Read the model definition and answer for the solid it produces. Units are mm, in the model's axes. A direction names the side the tool comes from. Give positions to 0.01 mm unless a question says otherwise; leave off trailing zeros. Order: outer loops, then holes, each group sorted by start corner. A loop starts at its lowest first (then second) coordinate and runs counter-clockwise, first axis right, second up.
```python
from build123d import *

# Parameters (mm, degrees)
SKETCH_W        = 56
SKETCH_H        = 45
PAD_DEPTH       = 1
SKETCH001_W     = 53
SKETCH001_H     = 34
PAD001_DEPTH    = 2
SKETCH002_W     = 10
SKETCH002_H     = 5
PAD002_DEPTH    = 4
SKETCH003_R     = 1.7
POCKET_DEPTH    = 38.501
SKETCH004_W     = 6
SKETCH004_H     = 3
POCKET001_DEPTH = 6
FILLET_R        = 4


with BuildPart() as part:
    # Sketch → Pad (new body, symmetric)
    with BuildSketch(Plane.XY):
        with Locations((28, 22.5)):
            Rectangle(SKETCH_W, SKETCH_H)
    extrude(amount=PAD_DEPTH, both=True)

    # Sketch001 (on Face6 of Pad) → Pad001 (join)
    with BuildSketch(Plane.XY.offset(1)):
        with Locations((28, 23.5)):
            Rectangle(SKETCH001_W, SKETCH001_H)
    extrude(amount=PAD001_DEPTH)

    # Sketch002 (on Face11 of Pad001) → Pad002 (join)
    with BuildSketch(Plane.XY.offset(3)):
        with Locations((28, 9)):
            Rectangle(SKETCH002_W, SKETCH002_H)
    extrude(amount=PAD002_DEPTH)

    # Sketch003 (on Face12 of Pad002) → Pocket (cut, through all)
    with BuildSketch(Plane.XZ.offset(-6.5)):
        with Locations((28, 4)):
            Circle(SKETCH003_R)
    extrude(amount=-POCKET_DEPTH, mode=Mode.SUBTRACT)

    # Sketch004 → Pocket001 (cut)
    with BuildSketch(Plane.XY.offset(7)):
        with Locations((28, 9)):
            Rectangle(SKETCH004_W, SKETCH004_H)
    extrude(amount=-POCKET001_DEPTH, mode=Mode.SUBTRACT)

    # Fillet
    fillet_edges = [part.edges().sort_by_distance(p)[0] for p in [
        (0, 0, 0),
        (56, 0, 0),
    ]]
    fillet(fillet_edges, radius=FILLET_R)


solid = part.part
```
1) For a pull along Y with two mould halves and no side action, classify faces 4 (the face through (28, 7, 7)), 5 (the face through (28, 45, 0)), 6 (the face through (28, 9, 1)) as released by +Y, released by -Y, zero draft, split by the parting line, or undercut.
Final values:
face 4: zero draft
face 5: released by +Y
face 6: undercut
2) The part is cut by section C-C on x = 5. Determine the outline of the cut face in (y, z).
Final values:
outline: (0, -1) - (45, -1) - (45, 1) - (40.5, 1) - (40.5, 3) - (6.5, 3) - (6.5, 1) - (0, 1) - close
3) Given pin 1 (2 mm diameter, centred on y = 8.5, z = 4.5, fed in from +X); pin 2 (1.2 mm diameter, centred on x = 28.5, z = 6, fed in from +Y); pin 3 (1.8 mm diameter, centred on x = 32, z = 2.5, fed in from -Y), each flat-ended and moving along its own axis, determine where each tip first touches the part or whether it passes through.
Final values:
pin 1: stops at x = 33
pin 2: stops at y = 11.5
pin 3: stops at y = 6.5
4) The part is cut by section B-B on z = 4. Determine the outline of the cut face in (x, y).
Final values:
outline: (23, 6.5) - (26.3, 6.5) - (26.3, 7.5) - (25, 7.5) - (25, 10.5) - (26.3, 10.5) - (26.3, 11.5) - (23, 11.5) - close; (29.7, 6.5) - (33, 6.5) - (33, 11.5) - (29.7, 11.5) - (29.7, 10.5) - (31, 10.5) - (31, 7.5) - (29.7, 7.5) - close
5) Consider L1, parallel to Z at x = 28, y = 7; L2, parallel to X at y = 9, z = 3.75; L3, parallel to X at y = 11.5, z = 1.75. Determine where each line is inside the solid, lowest interval first.
Final values:
L1: z = -1 to 2.3, 5.7 to 7
L2: x = 23 to 25, 31 to 33
L3: x = 1.5 to 54.5
6) The part is cut by section D-D on y = 37. Determine the outline of the cut face in (x, z).
Final values:
outline: (0, -1) - (56, -1) - (56, 1) - (54.5, 1) - (54.5, 3) - (29.37, 3) arc R1.7 cw to (26.63, 3) - (1.5, 3) - (1.5, 1) - (0, 1) - close
7) The part is cut by section A-A on x = 28. Determine the outline of the cut face in (y, z).
Final values:
outline: (0, -1) - (45, -1) - (45, 1) - (40.5, 1) - (40.5, 2.3) - (10.5, 2.3) - (10.5, 1) - (7.5, 1) - (7.5, 2.3) - (6.5, 2.3) - (6.5, 1) - (0, 1) - close; (6.5, 5.7) - (7.5, 5.7) - (7.5, 7) - (6.5, 7) - close; (10.5, 5.7) - (11.5, 5.7) - (11.5, 7) - (10.5, 7) - close
8) A tool of negligible diameter and unlimited length cuts with its end or side. For faces 1 (the face through (28, 6.5, 2)), 2 (the face through (28, 40.5, 2)), 3 (the face through (29.3, 7.5, 5.4)), from which of +Z, -Z, +X, -X, +Y, -Y can it reach the whole face along a straight path? Write none if from no direction.
Final values:
face 1: +Z, +X, -X, -Y
face 2: +Z, +X, -X, +Y
face 3: +Z
